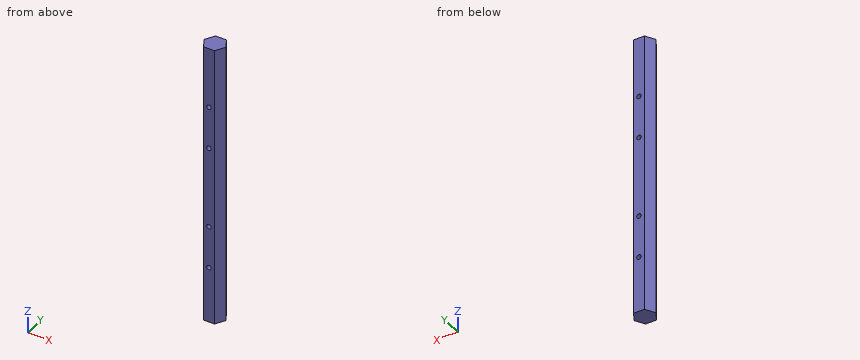
Autodesk Inventor part; units mm, degrees
ref_plane "YZ Plane" through (0, 0, 0) normal (1, 0, 0) x (0, 1, 0)
ref_plane "XZ Plane" through (0, 0, 0) normal (0, 1, 0) x (-1, 0, 0)
ref_plane "XY Plane" through (0, 0, 0) normal (0, 0, 1) x (1, 0, 0)
sketch "Sketch4" plane through (0, 0, 0) normal (0, 0, 1) x (1, 0, 0)
  line L0 (0, 0) -> (3.1, 0) construction
  circle A0 centre (0, 0) radius 3.1 construction
  line L1 (0, 0) -> (1.55, 2.6847) construction
  line L2 (0, 0) -> (-1.55, 2.6847) construction
  line L3 (0, 0) -> (-3.1, 0) construction
  line L4 (0, 0) -> (-1.55, -2.6847) construction
  line L5 (0, 0) -> (1.55, -2.6847) construction
  line L6 (-1.55, 2.6847) -> (1.55, 2.6847)
  line L7 (1.55, 2.6847) -> (3.1, 0)
  line L8 (3.1, 0) -> (1.55, -2.6847)
  line L9 (1.55, -2.6847) -> (-1.55, -2.6847)
  line L10 (-1.55, -2.6847) -> (-3.1, 0)
  line L11 (-3.1, 0) -> (-1.55, 2.6847)
  dimension "d15" = 3.1
  dimension "d18" = 360
extrude "Extrusion5" add sketch "Sketch4" along normal blind 80
sketch "Sketch5" plane through (-1.55, 2.6847, 0) normal (0, 1, 0) x (1, 0, 0)
  line L0 (3.1, -80) -> (0, -80) construction
  line L1 (3.1, 0) -> (0, 0) construction
  line L2 (0, -80) -> (3.1, -80)
  line L3 (1.55, -80) -> (1.55, 0) construction
  circle A0 centre (1.55, -15.9) radius 0.65
  circle A1 centre (1.55, -27.9) radius 0.65
  circle A2 centre (1.55, -50.9) radius 0.65
  circle A3 centre (1.55, -62.9) radius 0.65
  dimension "d22" = 1.3
  dimension "d23" = 64.1
  dimension "d24" = 52.1
  dimension "d25" = 29.1
  dimension "d26" = 17.1
extrude "Extrusion6" cut sketch "Sketch5" against normal blind 6
properties part number "Eje1"
The model under review builds one solid part; all positions refer to its coordinate system, in mm. Round coordinates to 2 decimals unless told otherwise and drop trailing zeros. Loops run counter-clockwise (first coordinate to the right, second up) from the corner with the lowest first, then second, coordinate; pieces in that order, holes last. Notation, with made-up numbers: (88.5, 41.5) -> (101.5, 41.5) arc R17 ccw to (101.5, 55.5) -> close; hole circle Ø10 at (-15, 69). An arc over 180 degrees is marked (long way). One line per question, with ' | ' between items. Start each with the question number.
Item 1: Add section B-B, the plane x = 0. Write out the cut boundary in (y, z), then the cut area to 3 significant figures.
Item 2: Add section A-A, the plane z = 27.9. Write out the cut boundary in (x, y), then the cut area to 3 significant figures.
Item 3: For pin 1 (3 mm diameter, centred on y = 1, z = 33, fed in from +X), flat-tipped, find the tip position at first contact; note if it passes through.
Item 4: Add section C-C, the plane y = 1.4. Write out the cut boundary in (x, z), then the cut area to 3 significant figures.
Item 5: Wall thickness on line 1 along Z through (x, y) = (0, 1); line 2 along X through (y, z) = (-1.4, 62.9); line 3 along Z through (x, y) = (-0.5, 0.5): over which ranges is each line inside the solid? List them lowest first. Write a range as [from, to].
Return value:
1) outline: (-2.68, 0) -> (2.68, 0) -> (2.68, 15.25) -> (-2.68, 15.25) -> close; (-2.68, 16.55) -> (2.68, 16.55) -> (2.68, 27.25) -> (-2.68, 27.25) -> close; (-2.68, 28.55) -> (2.68, 28.55) -> (2.68, 50.25) -> (-2.68, 50.25) -> close; (-2.68, 51.55) -> (2.68, 51.55) -> (2.68, 62.25) -> (-2.68, 62.25) -> close; (-2.68, 63.55) -> (2.68, 63.55) -> (2.68, 80) -> (-2.68, 80) -> close | area: 402 mm2
2) outline: (-3.1, 0) -> (-1.55, -2.68) -> (-0.65, -2.68) -> (-0.65, 2.68) -> (-1.55, 2.68) -> close; (0.65, -2.68) -> (1.55, -2.68) -> (3.1, 0) -> (1.55, 2.68) -> (0.65, 2.68) -> close | area: 18.0 mm2
3) pin 1: stops at x = 3.1
4) outline: (-2.29, 0) -> (2.29, 0) -> (2.29, 80) -> (-2.29, 80) -> close; hole circle Ø1.3 at (0, 15.9); hole circle Ø1.3 at (0, 27.9); hole circle Ø1.3 at (0, 50.9); hole circle Ø1.3 at (0, 62.9) | area: 361 mm2
5) line 1: z = [0, 15.25], [16.55, 27.25], [28.55, 50.25], [51.55, 62.25], [63.55, 80] | line 2: x = [-2.29, -0.65], [0.65, 2.29] | line 3: z = [0, 15.48], [16.32, 27.48], [28.32, 50.48], [51.32, 62.48], [63.32, 80]
